The model under review builds one solid part; all positions refer to its coordinate system, in mm. Face numbers are marked on the shaded views. A direction names the side the tool comes from. Round coordinates to 2 decimals unless told otherwise and drop trailing zeros. Order: outer loops, then holes, each group sorted by start corner. A loop starts at its lowest first (then second) coordinate and runs counter-clockwise, first axis right, second up. Notation, with made-up numbers: M 83,20.25 L 110,20.25 A32 ccw 110,58.25 Z; hole C 78.25,-6.5 d8. An arc over 180 degrees is marked long. Answer as a JSON object with one key per item and string values. Group by question number.
1) The part is to be moulded in two halves that separate along X. For the marked faces 3, 4 and 5, say which applies: +X half, -X half, draft (parallel to the pull), parting line (faces both ways), or undercut.
2) For the marked faces 1 and 2, list the 3-axis set-ups (+Z, -Z, +X, -X, +Y, -Y) from which the entire face can be reached by the end or side of a thin tool; tool diameter is ignored.
3) Consider section C-C, the plane y = 1. Write out the cut boundary in (x, z).
4) Consider section D-D, the plane y = 12.25. Write out the cut boundary in (x, z).
5) To check wall thickness, follow line 1 (X direction, y = 2.4, z = 0); line 2 (X direction, y = 10.05, z = 0); line 3 (Y direction, x = 9.5, z = 13). State the ranges of each line that lie inside material, in increasing order.
6) Insertion check: pin 1 Ø5.5 at (x, z) = (0.5, 0.5) entering from -Y; pin 2 Ø10.5 at (x, z) = (-8, -0.5) entering from +Y; pin 3 Ø1 at (y, z) = (6.5, 14.5) entering from +X; pin 4 Ø1.5 at (y, z) = (4.5, 3) entering from +X. Each pin has a flat end and moves straight along its axis. Give the tip position at first contact, or say it passes through.
```python
from build123d import *

# Parameters (mm, degrees)
SKETCH1_R           = 20
SKETCH1_R_2         = 17.5
BOSS_EXTRUDE1_DEPTH = 10
SKETCH2_R           = 17.5
BOSS_EXTRUDE3_DEPTH = 9.99
SKETCH4_R           = 2.5
BOSS_EXTRUDE4_DEPTH = 5
SKETCH3_R           = 2.5
CUT_EXTRUDE2_DEPTH  = 5


with BuildPart() as part:
    # Sketch1 → Boss-Extrude1 (new body)
    with BuildSketch(Plane(origin=(0, 0, 0), x_dir=(1, 0, 0), z_dir=(0, 1, 0))):
        with Locations(Location((0, 0, 0), (0, 0, 270))):
            Circle(SKETCH1_R)
        with Locations(Location((0, 0, 0), (0, 0, 270))):
            Circle(SKETCH1_R_2, mode=Mode.SUBTRACT)
    extrude(amount=BOSS_EXTRUDE1_DEPTH)



with BuildPart() as body_2:
    # Sketch2 → Boss-Extrude3 (new body)
    with BuildSketch(Plane(origin=(0, 0, 0), x_dir=(1, 0, 0), z_dir=(0, 1, 0))):
        with Locations(Location((0, 0, 0), (0, 0, 270))):
            Circle(SKETCH2_R)
    extrude(amount=BOSS_EXTRUDE3_DEPTH)


with BuildPart() as part_1:
    add(part.part)

    add(body_2.part)  # Boss-Extrude4 merges body 2
    # Sketch4 → Boss-Extrude4 (add)
    with BuildSketch(Plane(origin=(0, 9.99, 0), x_dir=(1, 0, 0), z_dir=(0, 1, 0))):
        with Locations(Location((0, 0, 0), (0, 0, 270))):
            Circle(SKETCH4_R)
    extrude(amount=BOSS_EXTRUDE4_DEPTH)

    # Sketch3 → Cut-Extrude2 (cut)
    with BuildSketch(Plane.XZ):
        with Locations(Location((0, 0, 0), (0, 0, 90))):
            Circle(SKETCH3_R)
    extrude(amount=-CUT_EXTRUDE2_DEPTH, mode=Mode.SUBTRACT)


solid = part_1.part
```
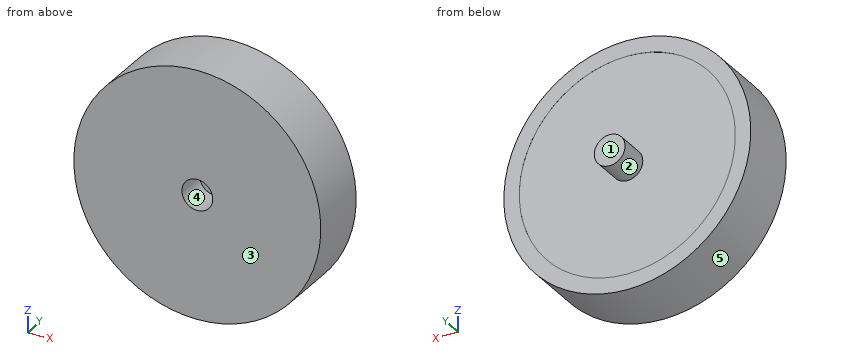
Results list:
{
 "1": {"face 3": "draft", "face 4": "undercut", "face 5": "parting line"},
 "2": {"face 1": "+Z, -Z, +X, -X, +Y", "face 2": "+Y"},
 "3": {"outline": "C 0,0 d40; hole C 0,0 d5"},
 "4": {"outline": "C 0,0 d5"},
 "5": {"line 1": "-20 to -2.5, 2.5 to 20", "line 2": "-2.5 to 2.5", "line 3": "0 to 9.99"},
 "6": {"pin 1": "y = 0", "pin 2": "y = 9.99", "pin 3": "x = 14.28", "pin 4": "x = 19.87"}
}
